For this review, take the finished solid that the model builds, in its own axes (mm). Give positions to 0.01 mm unless a question says otherwise; leave off trailing zeros. Order: outer loops, then holes, each group sorted by start corner. A loop starts at its lowest first (then second) coordinate and runs counter-clockwise, first axis right, second up.
Item 1: Consider section A-A (x = 0). Give the boundary of the cut face in (y, z) (3 decimals).
Item 2: Consider section C-C (y = 2.15). Give the number of separate pieces and of enclosed holes in the cut face, plus the area to 3 significant figures.
Item 3: Consider section B-B (z = 0). Give the boundary of the cut face in (x, y) (3 decimals), plus the area to 3 significant figures.
Item 4: For P1, Ø1.4, axis at y = 2.5, z = 20, coming from the -X side; P2, Ø0.5, axis at y = 2, z = -19, coming from the +X side; P3, Ø1.9, axis at x = 1, y = 2, coming from the -Z side, all flat-tipped, find the tip position at first contact; note any pin that passes through.
Item 5: For probe 1 along X at (y, z) = (2.8, 18) (3 decimals); probe 2 along X at (y, z) = (2.2, -1) (3 decimals); probe 3 along X at (y, z) = (0.65, 0), list the stretches that pass through material, from the lowest coordinate up.
```python
from build123d import *

# Parameters (mm, degrees)
SKETCH1_R           = 22.5
SKETCH1_R_2         = 16
BOSS_EXTRUDE1_DEPTH = 1.55
SKETCH2_W           = 5.05
SKETCH2_H           = 5.05
BOSS_EXTRUDE2_DEPTH = 1.75
CIRPATTERN1_COUNT   = 16


with BuildPart() as part:
    # Sketch1 → Boss-Extrude1 (new body)
    with BuildSketch(Plane(origin=(0, 0, 0), x_dir=(1, 0, 0), z_dir=(0, 1, 0))):
        Circle(SKETCH1_R)
        Circle(SKETCH1_R_2, mode=Mode.SUBTRACT)
    extrude(amount=BOSS_EXTRUDE1_DEPTH)

    # Sketch2 → Boss-Extrude2 (add)
    with BuildSketch(Plane(origin=(0, 1.55, 0), x_dir=(1, 0, 0), z_dir=(0, 1, 0))):
        with Locations((0, 18.95)):
            Rectangle(SKETCH2_W, SKETCH2_H)
    boss_extrude2 = extrude(amount=BOSS_EXTRUDE2_DEPTH)

    # CirPattern1: Boss-Extrude2 ×16 about axis
    cirpattern1_axis = Axis((0, 0, 0), (0, 1, 0))
    for i in range(1, CIRPATTERN1_COUNT):
        add(boss_extrude2.rotate(cirpattern1_axis, i * 360 / CIRPATTERN1_COUNT))


solid = part.part
```
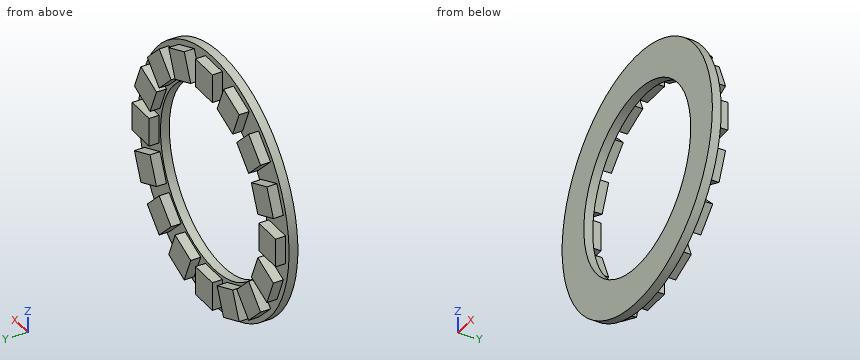
Resolved:
1. outline: (0, -22.5) - (1.55, -22.5) - (1.55, -21.475) - (3.3, -21.475) - (3.3, -16.425) - (1.55, -16.425) - (1.55, -16) - (0, -16) - close; (0, 16) - (1.55, 16) - (1.55, 16.425) - (3.3, 16.425) - (3.3, 21.475) - (1.55, 21.475) - (1.55, 22.5) - (0, 22.5) - close
2. separate pieces: 16
2. enclosed holes: 0
2. area: 408 mm2
3. outline: (-22.5, 0) - (-16, 0) - (-16, 1.55) - (-16.425, 1.55) - (-16.425, 3.3) - (-21.475, 3.3) - (-21.475, 1.55) - (-22.5, 1.55) - close; (16, 0) - (22.5, 0) - (22.5, 1.55) - (21.475, 1.55) - (21.475, 3.3) - (16.425, 3.3) - (16.425, 1.55) - (16, 1.55) - close
3. area: 37.8 mm2
4. P1: stops at x = -9.52
4. P2: stops at x = 10.55
4. P3: stops at z = -22.5
5. probe 1: x = -10.189 to -4.723, -2.525 to 2.525, 4.723 to 10.189
5. probe 2: x = -21.475 to -16.425, 16.425 to 21.475
5. probe 3: x = -22.5 to -16, 16 to 22.5
